Source: CAD feature listing. Evaluate the final solid. Frame: model axes, mm. Face numbers are marked on the shaded views. A direction names the side the tool comes from. Round coordinates to 2 decimals unless told otherwise and drop trailing zeros. Order: outer loops, then holes, each group sorted by start corner. A loop starts at its lowest first (then second) coordinate and runs counter-clockwise, first axis right, second up. Notation, with made-up numbers: (39, 56.25) - (50, 56.25) arc R27 ccw to (50, 93.25) - close; hole circle Ø2 at (10, 21.25). An arc over 180 degrees is marked (long way). Use one line per item in the form item = value. Start each with the question number.
Q1. Cut plane D-D, the plane y = -17.5. Return the cut outline in (x, z).
Q2. Ray query, line 1 (Z direction, x = -3, y = -15.5); line 2 (Z direction, x = -5, y = 12). Return the intervals inside material, ascending. Write a range as [from, to].
Q3. Draft query along Z for the marked faces 6, 7, 8 and 9. Return one class per face: released by +Z, released by -Z, zero draft, split by the parting line, or undercut.
Q4. Pin query (flat end, axial travel): pin 1 Ø8 at (y, z) = (12, 0) entering from -X; pin 2 Ø10 at (x, y) = (7, -9.5) entering from +Z; pin 3 Ø12 at (x, z) = (7, -0.5) entering from -Y; pin 4 Ø16 at (y, z) = (7, 4.5) entering from +X. Return the tip coordinate at first contact, or that it passes through.
Q5. Set-up query: the marked faces 1, 2, 3, 4 and 5. Return all of +Z, -Z, +X, -X, +Y, -Y with unobstructed straight access to the full face (end or side cutting, diameter ignored); none if empty.
Q6. Cut plane A-A, the plane y = 2.5. Return the cut outline in (x, z).
Q7. Cut plane C-C, the plane z = 12. Return the cut outline in (x, y), and give its area (3 significant figures).
Q8. Cut plane B-B, the plane x = 4. Return the cut outline in (y, z), and give its area (3 significant figures).
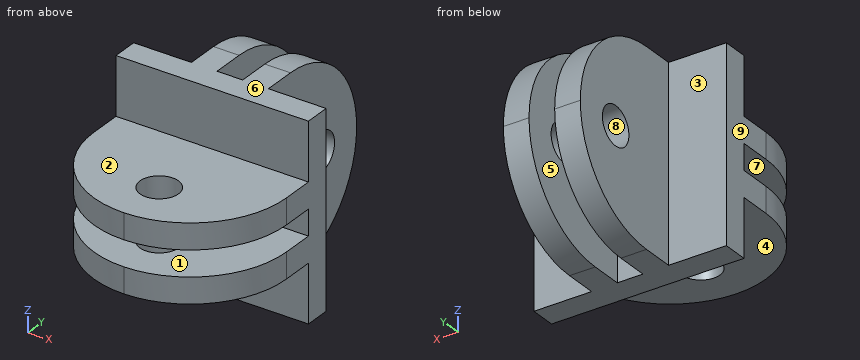
from build123d import *

# Parameters (mm, degrees)
F0_W      = 30
F0_H      = 30
F1_DEPTH  = 4
F2_W      = 4
F2_H      = 30
F3_DEPTH  = 20
F5_DEPTH  = 25
F6_R      = 3
F7_DEPTH  = 25
F8_W      = 30
F8_H      = 4
F9_DEPTH  = 20
F11_DEPTH = 25
F12_R     = 3
F13_DEPTH = 25


with BuildPart() as f1:
    # F0 (on Front) → F1 (new body)
    with BuildSketch(Plane.XZ):
        Rectangle(F0_W, F0_H)
    extrude(amount=F1_DEPTH)

    # F2 (on face) → F3 (join)
    with BuildSketch(Plane(origin=(0, 0, 0), x_dir=(-1, 0, 0), z_dir=(0, 1, 0))):
        with Locations((4, 0)):
            Rectangle(F2_W, F2_H)
        with Locations((-4, 0)):
            Rectangle(F2_W, F2_H)
    extrude(amount=F3_DEPTH)

    # F4 (on face) → F5 (cut)
    with BuildSketch(Plane(origin=(-6, 0, 0), x_dir=(0, -1, 0), z_dir=(-1, 0, 0))):
        with BuildLine():
            ThreePointArc((-5, -15), (-15.606602, -10.606602), (-20, 0))
            Line((-20, 0), (-20, -15))
            Line((-20, -15), (-5, -15))
        make_face()
        with BuildLine():
            Line((-5, 15), (-20, 15))
            Line((-20, 15), (-20, 0))
            ThreePointArc((-20, 0), (-15.606602, 10.606602), (-5, 15))
        make_face()
    extrude(amount=-F5_DEPTH, mode=Mode.SUBTRACT)

    # F6 (on face) → F7 (cut)
    with BuildSketch(Plane(origin=(-6, 0, 0), x_dir=(0, -1, 0), z_dir=(-1, 0, 0))):
        with Locations((-12, 0)):
            Circle(F6_R)
    extrude(amount=-F7_DEPTH, mode=Mode.SUBTRACT)

    # F8 (on face) → F9 (join)
    with BuildSketch(Plane.XZ.offset(4)):
        with Locations((0, 4)):
            Rectangle(F8_W, F8_H)
        with Locations((0, -4)):
            Rectangle(F8_W, F8_H)
    extrude(amount=F9_DEPTH)

    # F10 (on face) → F11 (cut)
    with BuildSketch(Plane.XY.offset(6)):
        with BuildLine():
            Line((-15, -24), (0, -24))
            ThreePointArc((0, -24), (-10.606602, -19.606602), (-15, -9))
            Line((-15, -9), (-15, -24))
        make_face()
        with BuildLine():
            ThreePointArc((15, -9), (10.606602, -19.606602), (0, -24))
            Line((0, -24), (15, -24))
            Line((15, -24), (15, -9))
        make_face()
    extrude(amount=-F11_DEPTH, mode=Mode.SUBTRACT)

    # F12 (on face) → F13 (cut)
    with BuildSketch(Plane.XY.offset(6)):
        with Locations((0, -16)):
            Circle(F12_R)
    extrude(amount=-F13_DEPTH, mode=Mode.SUBTRACT)


solid = f1.part
Completed:
q1.outline = (-12.36, -6) - (-2.6, -6) - (-2.6, -2) - (-12.36, -2) - close; (-12.36, 2) - (-2.6, 2) - (-2.6, 6) - (-12.36, 6) - close; (2.6, -6) - (12.36, -6) - (12.36, -2) - (2.6, -2) - close; (2.6, 2) - (12.36, 2) - (12.36, 6) - (2.6, 6) - close
q2.line_1 = [-6, -2], [2, 6]
q2.line_2 = [-13.27, -3], [3, 13.27]
q3.face_6 = released by +Z
q3.face_7 = undercut
q3.face_8 = undercut
q3.face_9 = zero draft
q4.pin_1 = -6
q4.pin_2 = 6
q4.pin_3 = -23.95
q4.pin_4 = 15
q5.face_1 = +X, -X, -Y
q5.face_2 = +Z, +X, -X, -Y
q5.face_3 = +Z, -Z, -X, +Y
q5.face_4 = -Z, +X, -X, -Y
q5.face_5 = +Z, -Z, +Y
q6.outline = (-6, -15) - (-2, -15) - (-2, 15) - (-6, 15) - close; (2, -15) - (6, -15) - (6, 15) - (2, 15) - close
q7.outline = (-15, -4) - (15, -4) - (15, 0) - (6, 0) - (6, 14) - (2, 14) - (2, 0) - (-2, 0) - (-2, 14) - (-6, 14) - (-6, 0) - (-15, 0) - close
q7.area = 232 mm2
q8.outline = (-23.46, -6) - (-4, -6) - (-4, -15) - (5, -15) arc R15 ccw to (20, 0) arc R15 ccw to (5, 15) - (-4, 15) - (-4, 6) - (-23.46, 6) - (-23.46, 2) - (-4, 2) - (-4, -2) - (-23.46, -2) - close; hole circle Ø6 at (12, 0)
q8.area = 751 mm2
